Part model, mm, in its own coordinate system. Face numbers are marked on the shaded views. A direction names the side the tool comes from. Round coordinates to 2 decimals unless told otherwise and drop trailing zeros. Loops run counter-clockwise (first coordinate to the right, second up) from the corner with the lowest first, then second, coordinate; pieces in that order, holes last. Notation, with made-up numbers: (26.5, -34) -> (55.5, -34) arc R18 ccw to (55.5, -16) -> close; hole circle Ø6 at (89.25, -35.75). An arc over 180 degrees is marked (long way). Answer as CSV lines item,"result".
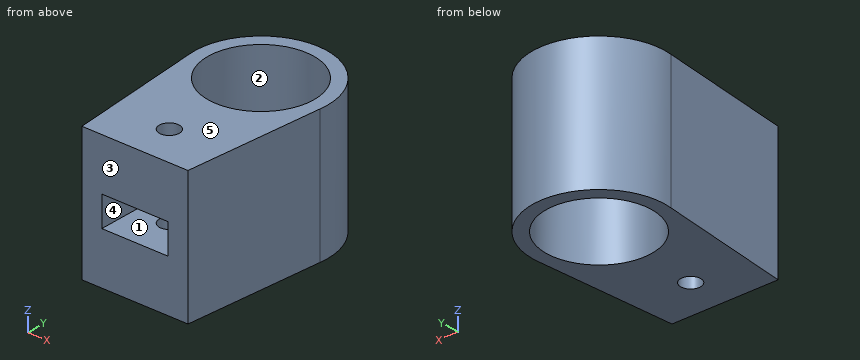
from build123d import *

# Parameters (mm, degrees)
SKETCH1_R           = 7.94
BOSS_EXTRUDE1_DEPTH = 10
BOSS_EXTRUDE2_START = 2.25
SKETCH1_3_W         = 10
SKETCH1_3_H         = 10
SKETCH1_3_R         = 1.5
BOSS_EXTRUDE2_DEPTH = 7.75


with BuildPart() as part:
    # Sketch1 → Boss-Extrude1 (new body)
    with BuildSketch(Plane.XY):
        with BuildLine():
            Line((8, -22), (9.871863704, -1.161854982))
            ThreePointArc((9.871863704, -1.161854982), (0, 9.94), (-9.871863704, -1.161854982))
            Line((-9.871863704, -1.161854982), (-8, -22))
            Line((-8, -22), (-5, -22))
            Line((-5, -22), (-5, -12))
            Line((-5, -12), (5, -12))
            Line((5, -12), (5, -22))
            Line((5, -22), (8, -22))
        make_face()
        Circle(SKETCH1_R, mode=Mode.SUBTRACT)
    extrude(amount=BOSS_EXTRUDE1_DEPTH)

    # Sketch1<3> → Boss-Extrude2 (add)
    with BuildSketch(Plane.XY.offset(BOSS_EXTRUDE2_START)):
        with Locations((0, -17)):
            Rectangle(SKETCH1_3_W, SKETCH1_3_H)
        with Locations((0, -16)):
            Circle(SKETCH1_3_R, mode=Mode.SUBTRACT)
    extrude(amount=BOSS_EXTRUDE2_DEPTH)

    # Mirror1: part across plane


with BuildPart() as part_1:
    add(part.part)
    add(part.part.mirror(Plane.XY))


solid = part_1.part
Q1. Two-plate mould, pull along Z, no slides. Class the marked faces 3, 4 and 5: pulls with the +Z half, pulls with the -Z half, needs draft (parallel to the pull), parting line crosses it, or undercut.
Geometry results:
face 3,"needs draft"
face 4,"undercut"
face 5,"pulls with the +Z half"
Q2. Which spindle directions (+Z, -Z, +X, -X, +Y, -Y) get a long thin tool onto all of the face, cutting with end or side? Do the marked faces 1 and 2. Say none if no direction does.
Geometry results:
face 1,"-Y"
face 2,"+Z, -Z"
Q3. Saw through at A-A, the plane x = 0. Write the cut outline in (y, z).
Geometry results:
outline,"(-22, -10) -> (-17.5, -10) -> (-17.5, -2.25) -> (-22, -2.25) -> close; (-22, 2.25) -> (-17.5, 2.25) -> (-17.5, 10) -> (-22, 10) -> close; (-14.5, -10) -> (-7.94, -10) -> (-7.94, 10) -> (-14.5, 10) -> (-14.5, 2.25) -> (-12, 2.25) -> (-12, -2.25) -> (-14.5, -2.25) -> close; (7.94, -10) -> (9.94, -10) -> (9.94, 10) -> (7.94, 10) -> close"
Q4. Drill centre lines: line 1 along Y through (x, z) = (0, 3.75); line 2 along Z through (x, y) = (-3.25, -19.5); line 3 along Y through (x, z) = (-0.75, -6). Where is each one in solid material? Low to high.
Geometry results:
line 1,"-22 to -17.5, -14.5 to -7.94, 7.94 to 9.94"
line 2,"-10 to -2.25, 2.25 to 10"
line 3,"-22 to -17.3, -14.7 to -7.9, 7.9 to 9.91"
Q5. Drop flat-ended pins along their axis: P1, Ø1.5, axis at x = 1, y = 6.5, coming from the -Z side; P2, Ø8, axis at y = -16, z = 5, coming from the -X side; P3, Ø6, axis at y = -13.5, z = -7, coming from the -X side; P4, Ø1.3, axis at y = -17.5, z = 1, coming from the +X side. Give the stop position or say it passes through.
Geometry results:
P1,"through"
P2,"x = -8.9"
P3,"x = -9.03"
P4,"x = 8.46"
Q6. Saw through at B-B, the plane z = 6.5. Write the cut outline in (x, y), then the cut area to 3 significant figures.
Geometry results:
outline,"(-9.87, -1.16) -> (-8, -22) -> (8, -22) -> (9.87, -1.16) arc R9.94 ccw (long way) to start; hole circle Ø15.88 at (0, 0); hole circle Ø3 at (0, -16)"
area,"346 mm2"
Q7. Saw through at D-D, the plane y = 2.5. Write the cut outline in (x, z), then the cut area to 3 significant figures.
Geometry results:
outline,"(-9.62, -10) -> (-7.54, -10) -> (-7.54, 10) -> (-9.62, 10) -> close; (7.54, -10) -> (9.62, -10) -> (9.62, 10) -> (7.54, 10) -> close"
area,"83.4 mm2"
Q8. Saw through at C-C, the plane x = -2.25. Write the cut outline in (y, z).
Geometry results:
outline,"(-22, -10) -> (-7.61, -10) -> (-7.61, 10) -> (-22, 10) -> (-22, 2.25) -> (-12, 2.25) -> (-12, -2.25) -> (-22, -2.25) -> close; (7.61, -10) -> (9.68, -10) -> (9.68, 10) -> (7.61, 10) -> close"
